from build123d import *

# Parameters (mm, degrees)
ESQUISSE2_R      = 1
EXTRUSION1_DEPTH = 7


with BuildPart() as part:
    # Esquisse1 → Révolution1 (revolve)
    with BuildSketch(Plane.XY, mode=Mode.PRIVATE) as r_volution1_sk:
        with BuildLine():
            Line((0, 0), (4, 0))
            Line((4, 0), (3.5, 55))
            Line((3.5, 55), (2.5, 55))
            Line((2.5, 55), (2.5, 55.5))
            Line((2.5, 55.5), (3.495454545, 55.5))
            Line((3.495454545, 55.5), (3.486363636, 56.5))
            Line((3.486363636, 56.5), (2.486363636, 56.5))
            Line((2.486363636, 56.5), (2.486363636, 57))
            Line((2.486363636, 57), (3.481818182, 57))
            Line((3.481818182, 57), (3.440081364, 61.591049954))
            ThreePointArc((3.440081364, 61.591049954), (2.421523292, 64.003413687), (0, 65))
            Line((0, 65), (0, 0))
        make_face()
    revolve(r_volution1_sk.sketch.rotate(Axis((0, 0, 0), (0, 1, 0)), 90), axis=Axis((0, 0, 0), (0, 1, 0)))

    # Esquisse2 → Extrusion1 (add, symmetric)
    with BuildSketch(Plane.XY):
        with Locations(Location((0, 2, 0), (0, 0, 222.556975448))):
            Circle(ESQUISSE2_R)
    extrude(amount=EXTRUSION1_DEPTH, both=True)


solid = part.part
Source: CAD feature listing. Evaluate the final solid. Frame: model axes, mm. A direction names the side the tool comes from. Round coordinates to 2 decimals unless told otherwise and drop trailing zeros. Loops run counter-clockwise (first coordinate to the right, second up) from the corner with the lowest first, then second, coordinate; pieces in that order, holes last. Notation, with made-up numbers: M 7,61.5 L 16,61.5 A21 ccw 16,97.5 Z; hole C 9.25,-9.5 d6. An arc over 180 degrees is marked long. Return JSON: item names as keys, results as strings. Group by question number.
1. Mould query, pull axis Y, two halves, no side actions, for faces 6 (the face through (2, 56.5, -2)), 7 (the face through (-1.05, 56.01, -3.33)), 8 (the face through (0, 2, -7)), 9 (the face through (2.3, 57, 1.5)). Classes: released by +Y, released by -Y, zero draft, split by the parting line, or undercut.
2. Section query A-A on y = 2. Output: boundary loops of the cut face in (x, z), and give its area (3 significant figures).
3. Reachability of faces 1 (the face through (-3.43, 59.33, 0.45)), 2 (the face through (0, 0, 0)), 3 (the face through (0, 1, 5)), 4 (the face through (0, 1, -5)), 5 (the face through (-0.75, 56.75, -2.37)) from +Z, -Z, +X, -X, +Y, -Y: full face, straight path, thin tool, end or side. Return the list, or none.
4. Section query B-B on z = 6. Output: boundary loops of the cut face in (x, y).
5. Pin query (flat end, axial travel): pin 1 (3 mm diameter, centred on y = 40.5, z = -4, fed in from +X); pin 2 (3 mm diameter, centred on y = 7.5, z = 3, fed in from -X); pin 3 (1.5 mm diameter, centred on x = 1, y = 27.5, fed in from +Z). Return the tip coordinate at first contact, or that it passes through.
6. Material intervals for line 1 along Z through (x, y) = (-1, 40); line 2 along Z through (x, y) = (-0.75, 31); line 3 along X through (y, z) = (4, -0.25), sorted ascending. Write a range as from..to.
7. Section query C-C on y = 40. Output: boundary loops of the cut face in (x, z).
Checks:
{
 "1": {"face 6": "undercut", "face 7": "released by +Y", "face 8": "zero draft", "face 9": "undercut"},
 "2": {"outline": "M -1,-7 L 1,-7 L 1,-3.85 A3.98 ccw 1,3.85 L 1,7 L -1,7 L -1,3.85 A3.98 ccw -1,-3.85 Z", "area": "62.1 mm²"},
 "3": {"face 1": "+Y", "face 2": "+Z, -Z, +X, -X, -Y", "face 3": "+Z", "face 4": "-Z", "face 5": "none"},
 "4": {"outline": "C 0,2 d2"},
 "5": {"pin 1": "stops at x = 2.63", "pin 2": "stops at x = -3.63", "pin 3": "stops at z = 3.74"},
 "6": {"line 1": "z = -3.5..3.5", "line 2": "z = -3.64..3.64", "line 3": "x = -3.96..3.96"},
 "7": {"outline": "C 0,0 d7.27"}
}
